Model file for the job. Use its own axes, mm. Round coordinates to 2 decimals unless told otherwise and drop trailing zeros. Order: outer loops, then holes, each group sorted by start corner. A loop starts at its lowest first (then second) coordinate and runs counter-clockwise, first axis right, second up. Notation, with made-up numbers: (42.5, 78) - (68.5, 78) arc R27 cw to (68.5, 98) - close; hole circle Ø2 at (78, 3). An arc over 180 degrees is marked (long way). Write item = value, one per line. Start each with the question number.
from build123d import *

# Parameters (mm, degrees)
EXTRUDE_1_DEPTH          = 1.5
CUT_EXTRUDE_1_DEPTH      = 132.278330276
CUT_EXTRUDE_1_DEPTH_BACK = 1.5
SKETCH_3_W               = 152
SKETCH_3_H               = 3
CUT_EXTRUDE_2_DEPTH      = 1


with BuildPart() as part:
    # Эскиз1 → Бобышка-Вытянуть1 (new, symmetric)
    with BuildSketch(Plane(origin=(0, 0, 0), x_dir=(1, 0, 0), z_dir=(0, 1, 0))):
        with BuildLine():
            Line((-80, 100), (80, 100))
            ThreePointArc((80, 100), (83.535533906, 98.535533906), (85, 95))
            Line((85, 95), (85, -95))
            ThreePointArc((85, -95), (83.535533906, -98.535533906), (80, -100))
            Line((80, -100), (-80, -100))
            ThreePointArc((-80, -100), (-83.535533906, -98.535533906), (-85, -95))
            Line((-85, -95), (-85, 95))
            ThreePointArc((-85, 95), (-83.535533906, 98.535533906), (-80, 100))
        make_face()
        with BuildLine():
            Line((10, 50), (10, -50))
            ThreePointArc((10, -50), (0, -60), (-10, -50))
            Line((-10, -50), (-10, 50))
            ThreePointArc((-10, 50), (0, 60), (10, 50))
        make_face(mode=Mode.SUBTRACT)
    extrude(amount=EXTRUDE_1_DEPTH, both=True)

    # Эскиз3 → Вырез-Вытянуть1 (cut, two sides: drawn at the far end of the back side and taken through both)
    with BuildSketch(Plane(origin=(0, 1.5, 0), x_dir=(1, 0, 0), z_dir=(0, 1, 0)).offset(-CUT_EXTRUDE_1_DEPTH_BACK)):
        with Locations((0, -3)):
            Rectangle(SKETCH_3_W, SKETCH_3_H)
    extrude(amount=CUT_EXTRUDE_1_DEPTH + CUT_EXTRUDE_1_DEPTH_BACK, mode=Mode.SUBTRACT)

    # Эскиз4 → Вырез-Вытянуть2 (cut)
    with BuildSketch(Plane(origin=(0, 1.5, 0), x_dir=(1, 0, 0), z_dir=(0, 1, 0))):
        with BuildLine():
            Line((88.228937258, -1.5), (-88.228937258, -1.5))
            ThreePointArc((-88.228937258, -1.5), (-89.728937258, 0), (-88.228937258, 1.5))
            Line((-88.228937258, 1.5), (88.228937258, 1.5))
            ThreePointArc((88.228937258, 1.5), (89.728937258, 0), (88.228937258, -1.5))
        make_face()
    extrude(amount=-CUT_EXTRUDE_2_DEPTH, mode=Mode.SUBTRACT)


solid = part.part
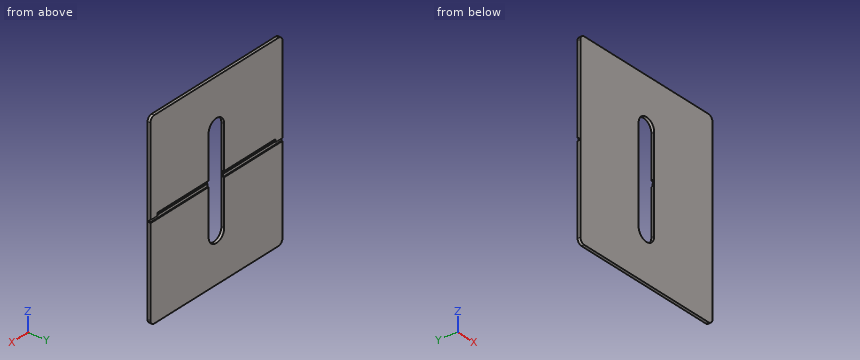
Item 1: Saw through at C-C, the plane x = 0. Give the cut face in (y, z).
Item 2: Saw through at B-B, the plane z = -11.5. Give the cut face in (x, y).
Item 3: Drop flat-ended pins along their axis: pin 1 (1.5 mm diameter, centred on x = -32, z = 0, fed in from +Y); pin 2 (0.9 mm diameter, centred on x = -58.5, z = 3, fed in from +Y); pin 3 (0.5 mm diameter, centred on x = -82, y = 1, fed in from -Z). Give the stop position or say it passes through.
Item 4: Probe L1, parallel to X at y = 0.45, z = 6.5; L2, parallel to Z at x = 53, y = 1.25; L3, parallel to Z at x = -32, y = 0.35. List the from-to ranges inside material, lowest first.
Item 5: Saw through at A-A, the plane y = 1. Give the cut face in (x, z), then the cut area to 3 significant figures.
Check sheet entries:
q1.outline = (-1.5, -100) - (1.5, -100) - (1.5, -60) - (-1.5, -60) - close; (-1.5, 60) - (1.5, 60) - (1.5, 100) - (-1.5, 100) - close
q2.outline = (-85, -1.5) - (-10, -1.5) - (-10, 1.5) - (-85, 1.5) - close; (10, -1.5) - (85, -1.5) - (85, 1.5) - (10, 1.5) - close
q3.pin_1 = 0.5
q3.pin_2 = 0
q3.pin_3 = -99.68
q4.L1 = -85 to -10, 10 to 85
q4.L2 = -100 to -1.5, 4.5 to 100
q4.L3 = -100 to 1.5, 4.5 to 100
q5.outline = (-85, -95) arc R5 ccw to (-80, -100) - (80, -100) arc R5 ccw to (85, -95) - (85, -1.5) - (10, -1.5) - (10, -50) arc R10 cw to (-10, -50) - (-10, -1.5) - (-85, -1.5) - close; (-85, 1.5) - (-76, 1.5) - (-76, 4.5) - (-10, 4.5) - (-10, 50) arc R10 cw to (10, 50) - (10, 4.5) - (76, 4.5) - (76, 1.5) - (85, 1.5) - (85, 95) arc R5 ccw to (80, 100) - (-80, 100) arc R5 ccw to (-85, 95) - close
q5.area = 30,800 mm2
